Part print with two shaded views. Sizes in mm from the minimum x, y, z corner. Give positions to 0.01 mm unless a question says otherwise; leave off trailing zeros. Order: outer loops, then holes, each group sorted by start corner. A loop starts at its lowest first (then second) coordinate and runs counter-clockwise, first axis right, second up. Notation, with made-up numbers: (48, 80.25) - (88, 80.25) arc R15 cw to (88, 93.25) - close; hole circle Ø4 at (16, 63). An arc over 180 degrees is marked (long way). Return JSON: item names as keys, results as strings. Group by question number.
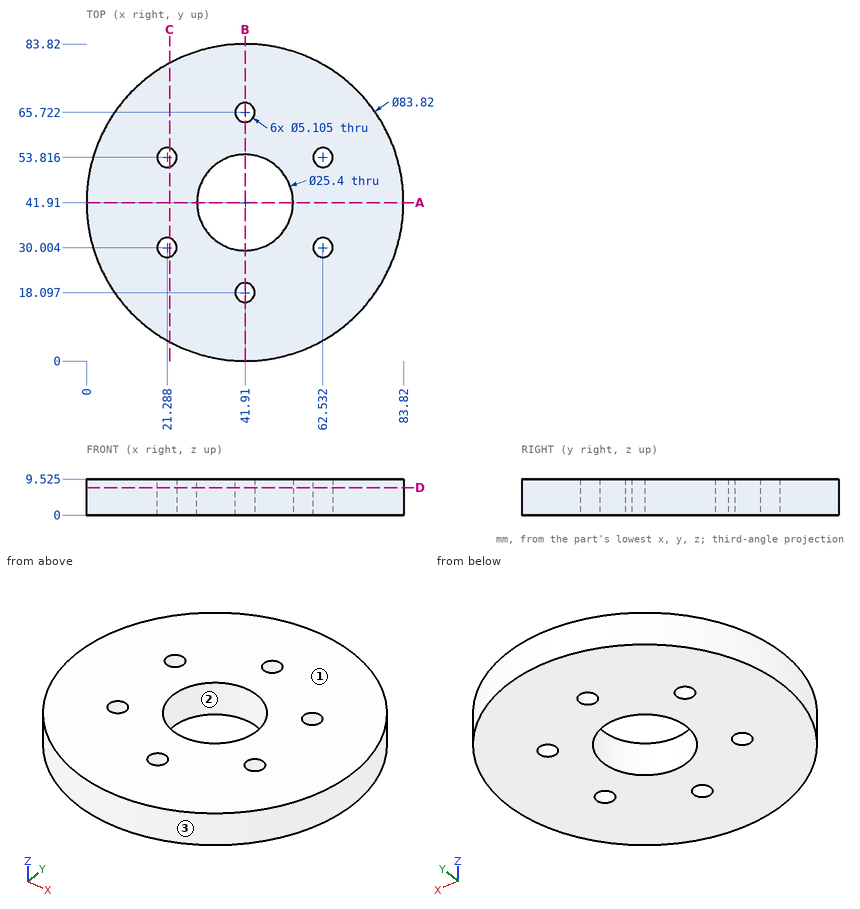
(1) Slice it at C-C (x = 22). Give the cut face in (y, z) (1 decimal), and give its area (3 significant figures).
(2) Drill centre lines: L1, parallel to X at y = 42.5, z = 7 (1 decimal); L2, parallel to Y at x = 64, z = 3 (1 decimal); L3, parallel to Y at x = 41, z = 8.25. Where is each one in solid material? Low to high.
(3) Pull direction Y, two halves, no side cores. Call the marked faces 1, 2 and 3: released by +Y, released by -Y, zero draft, split by the parting line, or undercut.
(4) Slice it at A-A (y = 41.91). Give the cut face in (x, z) (1 decimal).
(5) Slice it at B-B (x = 41.91). State how many separate pieces and enclosed holes the cut face has, and give its area (3 significant figures).
(6) Slice it at D-D (z = 7.25). Give the cut face in (x, y) (1 decimal), and give its area (3 significant figures).
(7) Drop flat-ended pins along their axis: pin 1 Ø1.5 at (y, z) = (47.5, 4.5) entering from +X; pin 2 Ø4.5 at (x, y) = (21.29, 53.82) entering from -Z; pin 3 Ø4 at (x, z) = (70, 5.5) entering from -Y; pin 4 Ø4 at (y, z) = (24.5, 4.5) entering from -X (1 decimal). Give the stop position or say it passes through.
Result set:
{
 "1": {"outline": "(5, 0) - (27.6, 0) - (27.6, 9.5) - (5, 9.5) - close; (32.5, 0) - (51.4, 0) - (51.4, 9.5) - (32.5, 9.5) - close; (56.3, 0) - (78.8, 0) - (78.8, 9.5) - (56.3, 9.5) - close", "area": "609 mm²"},
 "2": {"L1": "x = 0 to 29.2, 54.6 to 83.8", "L2": "y = 6.3 to 27.9, 32.1 to 51.7, 55.9 to 77.5", "L3": "y = 0.01 to 15.71, 20.48 to 29.24, 54.58 to 63.34, 68.11 to 83.81"},
 "3": {"face 1": "zero draft", "face 2": "undercut", "face 3": "split by the parting line"},
 "4": {"outline": "(0, 0) - (29.2, 0) - (29.2, 9.5) - (0, 9.5) - close; (54.6, 0) - (83.8, 0) - (83.8, 9.5) - (54.6, 9.5) - close"},
 "5": {"separate pieces": "4", "enclosed holes": "0", "area": "459 mm²"},
 "6": {"outline": "circle Ø83.8 at (41.9, 41.9); hole circle Ø5.1 at (21.3, 30); hole circle Ø5.1 at (21.3, 53.8); hole circle Ø25.4 at (41.9, 41.9); hole circle Ø5.1 at (41.9, 18.1); hole circle Ø5.1 at (41.9, 65.7); hole circle Ø5.1 at (62.5, 30); hole circle Ø5.1 at (62.5, 53.8)", "area": "4,890 mm²"},
 "7": {"pin 1": "stops at x = 83.54", "pin 2": "passes through", "pin 3": "stops at y = 9.11", "pin 4": "stops at x = 2.9"}
}
